from build123d import *

# Parameters (mm, degrees)
ESBO_O1_W                  = 390
ESBO_O1_H                  = 95
RESSALTO_EXTRUS_O1_DEPTH   = 9.525
ESBO_O3_R                  = 16
CIRCULO_DE_ROLAMENTO_DEPTH = 9.525
ESBO_O4_R                  = 2
CORTE_EXTRUS_O3_DEPTH      = 20
CORTE_EXTRUS_O4_START      = -20
ESBO_O5_R                  = 2
CORTE_EXTRUS_O4_DEPTH      = 20


with BuildPart() as part:
    # Esboço1 → Ressalto-extrusão1 (new body)
    with BuildSketch(Plane.XY):
        Rectangle(ESBO_O1_W, ESBO_O1_H)
    extrude(amount=RESSALTO_EXTRUS_O1_DEPTH)

    # Esboço3 → Circulo de rolamento (cut)
    with BuildSketch(Plane.XY.offset(9.525)):
        with Locations((-0.011971039, -8.12)):
            Circle(ESBO_O3_R)
    extrude(amount=-CIRCULO_DE_ROLAMENTO_DEPTH, mode=Mode.SUBTRACT)

    # Esboço4 → Corte-extrusão3 (cut)
    with BuildSketch(Plane(origin=(0, 47.5, 0), x_dir=(1, 0, 0), z_dir=(0, 1, 0))):
        with Locations(Location((175, -4.7625, 0), (0, 0, 270))):
            Circle(ESBO_O4_R)
        with Locations(Location((85, -4.7625, 0), (0, 0, 270))):
            Circle(ESBO_O4_R)
        with Locations(Location((0, -4.7625, 0), (0, 0, 270))):
            Circle(ESBO_O4_R)
        with Locations(Location((-175, -4.7625, 0), (0, 0, 90))):
            Circle(ESBO_O4_R)
        with Locations(Location((-85, -4.7625, 0), (0, 0, 90))):
            Circle(ESBO_O4_R)
    extrude(amount=-CORTE_EXTRUS_O3_DEPTH, mode=Mode.SUBTRACT)

    # Esboço5 → Corte-extrusão4 (cut)
    with BuildSketch(Plane.XZ.offset(47.5).offset(CORTE_EXTRUS_O4_START)):
        with Locations(Location((0, 4.7625, 0), (0, 0, 90))):
            Circle(ESBO_O5_R)
        with Locations(Location((-115, 4.7625, 0), (0, 0, 270))):
            Circle(ESBO_O5_R)
        with Locations(Location((115, 4.7625, 0), (0, 0, 270))):
            Circle(ESBO_O5_R)
    extrude(amount=CORTE_EXTRUS_O4_DEPTH, mode=Mode.SUBTRACT)


solid = part.part
Can you work these out from the model? Positions are in its coordinate system, mm. Coordinates: 2 decimals unless noted, no trailing zeros. Write each loop counter-clockwise with the first axis right and the second up, starting at its lowest first coordinate (ties: lowest second). Pieces come first, ordered by that corner, then holes. Notation, with made-up numbers: (21, 40) - (50, 40) arc R27 ccw to (50, 61) - close; hole circle Ø6 at (-12, -9). An arc over 180 degrees is marked (long way). Return JSON: item names as keys, results as strings. Group by question number.
Item 1: Please list where these lines run through material, in increasing order: probe 1 along X at (y, z) = (-28, 3.75); probe 2 along Z at (x, y) = (-175, 33) (1 decimal); probe 3 along X at (y, z) = (-9, 7.25).
Item 2: I'm going to push flat-ended pins straight in: pin 1 Ø6 at (x, y) = (-62.5, -12.5) entering from -Z; pin 2 Ø3 at (x, z) = (-175, 4.5) entering from +Y. Where does each tip first touch, or does it pass through?
Item 3: If we section it at A-A (y = -8.12): Write out the boundary of the cut face in (x, z) (3 decimals).
Item 4: We'd pull the mould along Y, two halves only. Please class faces 1 (the face through (-3, -47.5, 5)), 2 (the face through (15.25, -3.31, 4.83)), 3 (the face through (-3, 11, 9.525)): pulls with the +Y half, pulls with the -Y half, needs draft (parallel to the pull), parting line crosses it, or undercut.
Return value:
{
 "1": {"probe 1": "x = -195 to -116.72, -113.28 to -1.72, 1.72 to 113.28, 116.72 to 195", "probe 2": "z = 0 to 2.8, 6.8 to 9.5", "probe 3": "x = -195 to -15.99, 15.96 to 195"},
 "2": {"pin 1": "stops at z = 0", "pin 2": "stops at y = 27.5"},
 "3": {"outline": "(-195, 0) - (-16.012, 0) - (-16.012, 9.525) - (-195, 9.525) - close; (15.988, 0) - (195, 0) - (195, 9.525) - (15.988, 9.525) - close"},
 "4": {"face 1": "pulls with the -Y half", "face 2": "undercut", "face 3": "needs draft"}
}
